Verification items for the finished model (mm, model axes). A direction names the side the tool comes from. Give positions to 0.01 mm unless a question says otherwise; leave off trailing zeros. Order: outer loops, then holes, each group sorted by start corner. A loop starts at its lowest first (then second) coordinate and runs counter-clockwise, first axis right, second up. Notation, with made-up numbers: M -37.75,70 L -14.75,70 A15 ccw -14.75,92 Z; hole C 23.25,82 d6. An arc over 180 degrees is marked long. Answer as a JSON object with one key per item and string values.
```python
from build123d import *

# Parameters (mm, degrees)
F1_DEPTH = 2
F2_DEPTH = 0.6
F3_DEPTH = 5


with BuildPart() as f1:
    # F0 (on Right) → F1 (new body)
    with BuildSketch(Plane.YZ):
        with BuildLine():
            Line((-49.333436, 42.25241), (-47.034119, 46.923187))
            ThreePointArc((-47.034119, 46.923187), (-50.537652, 46.231209), (-53.82776, 44.842407))
            Line((-53.82776, 44.842407), (-50.170235, 40.552557))
            Line((-50.170235, 40.552557), (-49.333436, 42.25241))
        make_face()
        Polygon((-30.300626, 27.594882), (-28.371687, 33.48021), (-47.034119, 46.923187), (-49.333436, 42.25241), align=None)
        with BuildLine():
            ThreePointArc((-28.365389, 25.54377), (-28.026232, 27.508204), (-27.912688, 29.498465))
            ThreePointArc((-27.912688, 29.498465), (-28.027817, 31.502521), (-28.371687, 33.48021))
            Line((-28.371687, 33.48021), (-30.300626, 27.594882))
            Line((-30.300626, 27.594882), (-30.72083, 26.312811))
            Line((-30.72083, 26.312811), (-28.371687, 25.542871))
            Line((-28.371687, 25.542871), (-28.365389, 25.54377))
        make_face()
        with BuildLine():
            ThreePointArc((-28.371687, 33.48021), (-28.027817, 31.502521), (-27.912688, 29.498465))
            ThreePointArc((-27.912688, 29.498465), (-28.026232, 27.508204), (-28.365389, 25.54377))
            Line((-28.365389, 25.54377), (-26.486235, 25.812047))
            Line((-26.486235, 25.812047), (-25.734026, 26.853122))
            Line((-25.734026, 26.853122), (-26.24937, 32.784612))
            Line((-26.24937, 32.784612), (-28.371687, 33.48021))
        make_face()
        with BuildLine():
            ThreePointArc((-53.82776, 44.842407), (-50.537652, 46.231209), (-47.034119, 46.923187))
            Line((-47.034119, 46.923187), (-47.034119, 48.613626))
            Line((-47.034119, 48.613626), (-49.236418, 48.613626))
            Line((-49.236418, 48.613626), (-54.496467, 46.923187))
            Line((-54.496467, 46.923187), (-53.82776, 44.842407))
        make_face()
    extrude(amount=F1_DEPTH)

    # F0 (on Right) → F2 (cut)
    with BuildSketch(Plane.YZ):
        Polygon((-30.300626, 27.594882), (-28.371687, 33.48021), (-47.034119, 46.923187), (-49.333436, 42.25241), align=None)
    extrude(amount=F2_DEPTH, mode=Mode.SUBTRACT)

    # F0 (on Right) → F3 (join)
    with BuildSketch(Plane.YZ):
        with BuildLine():
            ThreePointArc((-53.82776, 44.842407), (-50.537652, 46.231209), (-47.034119, 46.923187))
            Line((-47.034119, 46.923187), (-47.034119, 48.613626))
            Line((-47.034119, 48.613626), (-49.236418, 48.613626))
            Line((-49.236418, 48.613626), (-54.496467, 46.923187))
            Line((-54.496467, 46.923187), (-53.82776, 44.842407))
        make_face()
        with BuildLine():
            ThreePointArc((-28.371687, 33.48021), (-28.027817, 31.502521), (-27.912688, 29.498465))
            ThreePointArc((-27.912688, 29.498465), (-28.026232, 27.508204), (-28.365389, 25.54377))
            Line((-28.365389, 25.54377), (-26.486235, 25.812047))
            Line((-26.486235, 25.812047), (-25.734026, 26.853122))
            Line((-25.734026, 26.853122), (-26.24937, 32.784612))
            Line((-26.24937, 32.784612), (-28.371687, 33.48021))
        make_face()
    extrude(amount=-F3_DEPTH)


solid = f1.part
```
Q1. Section check B-B on z = 31. Record the cut outline in (x, y), then the cut area to 3 significant figures.
Resolved:
{"outline": "M -5,-27.98 L 0,-27.98 L 0,-29.18 L 0.6,-29.18 L 0.6,-34.72 L 2,-34.72 L 2,-26.09 L -5,-26.09 Z", "area": "23.3 mm²"}
Q2. Material ranges on L1, parallel to X at y = -33.25, z = 30.25; L2, parallel to X at y = -48.25, z = 45.75; L3, parallel to Y at x = -3, z = 45.25, recorded low to high.
Resolved:
{"L1": "x = 0.6 to 2", "L2": "x = 0 to 2", "L3": "y = -53.96 to -53.04"}
Q3. Section check C-C on y = -47.5. Record the cut outline in (x, z), then the cut area to 3 significant figures.
Resolved:
{"outline": "M -5,46.87 L 0,46.87 L 0,45.98 L 0.6,45.98 L 0.6,40.84 L 2,40.84 L 2,48.61 L -5,48.61 Z", "area": "21.2 mm²"}
Q4. Section check D-D on z = 43.5. Record the cut outline in (x, y).
Resolved:
{"outline": "M 0,-52.68 L 2,-52.68 L 2,-42.28 L 0.6,-42.28 L 0.6,-48.72 L 0,-48.72 Z"}
Q5. Tool access check on faces 4 (the face through (-1.45, -51.83, 47.78)), 5 (the face through (0, -50, 44)), 6 (the face through (-1, -47.034, 48)), 7 (the face through (-2.465, -28.023, 27.536)). Record the directions out of +Z, -Z, +X, -X, +Y, -Y that give a thin tool (end or side, any length) a straight path to the whole face; none if there is none.
Resolved:
{"face 4": "+Z, +X, -X, -Y", "face 5": "-Z, -X, +Y", "face 6": "+Z, +X, -X, +Y", "face 7": "-X, -Y"}
Q6. Release check for a two-part mould opening along Y. For faces 1 (the face through (-1.55, -27.3, 33.13)), 2 (the face through (-5, -27, 30)), 3 (the face through (0.986, -29.563, 25.933)) record: +Y half, -Y half, draft (parallel to the pull), parting line (faces both ways), or undercut.
Resolved:
{"face 1": "+Y half", "face 2": "draft", "face 3": "-Y half"}
Q7. Section check A-A on x = -2. Record the cut outline in (y, z), then the cut area to 3 significant figures.
Resolved:
{"outline": "M -54.5,46.92 L -53.83,44.84 A17.5 cw -47.03,46.92 L -47.03,48.61 L -49.24,48.61 Z; M -28.37,25.54 L -26.49,25.81 L -25.73,26.85 L -26.25,32.78 L -28.37,33.48 A17.5 cw -27.91,29.5 A17.5 cw Z", "area": "29.2 mm²"}
Q8. Gauge pin test, flat ends, axial feed: pin 1 Ø0.5 at (x, z) = (-1.5, 48) entering from +Y; pin 2 Ø3 at (x, y) = (-1, -33.5) entering from +Z; pin 3 Ø2 at (y, z) = (-29, 30) entering from -X; pin 4 Ø4 at (y, z) = (-45, 38) entering from -X. Record the tip position at first contact, or that the pin passes through.
Resolved:
{"pin 1": "stops at y = -47.03", "pin 2": "passes through", "pin 3": "stops at x = 0", "pin 4": "stops at x = 0.6"}
